Can you work these out from the drawing? Everything is in mm from the part's minimum corner. Round coordinates to 2 decimals unless told otherwise and drop trailing zeros. Write each loop counter-clockwise with the first axis right and the second up, starting at its lowest first coordinate (ties: lowest second). Pieces come first, ordered by that corner, then holes. Notation, with made-up numbers: (21, 60) -> (52, 60) arc R26 cw to (52, 78) -> close; hole circle Ø2 at (55.25, 25.5). An arc over 180 degrees is marked (long way). Answer as CSV lines item,"result".
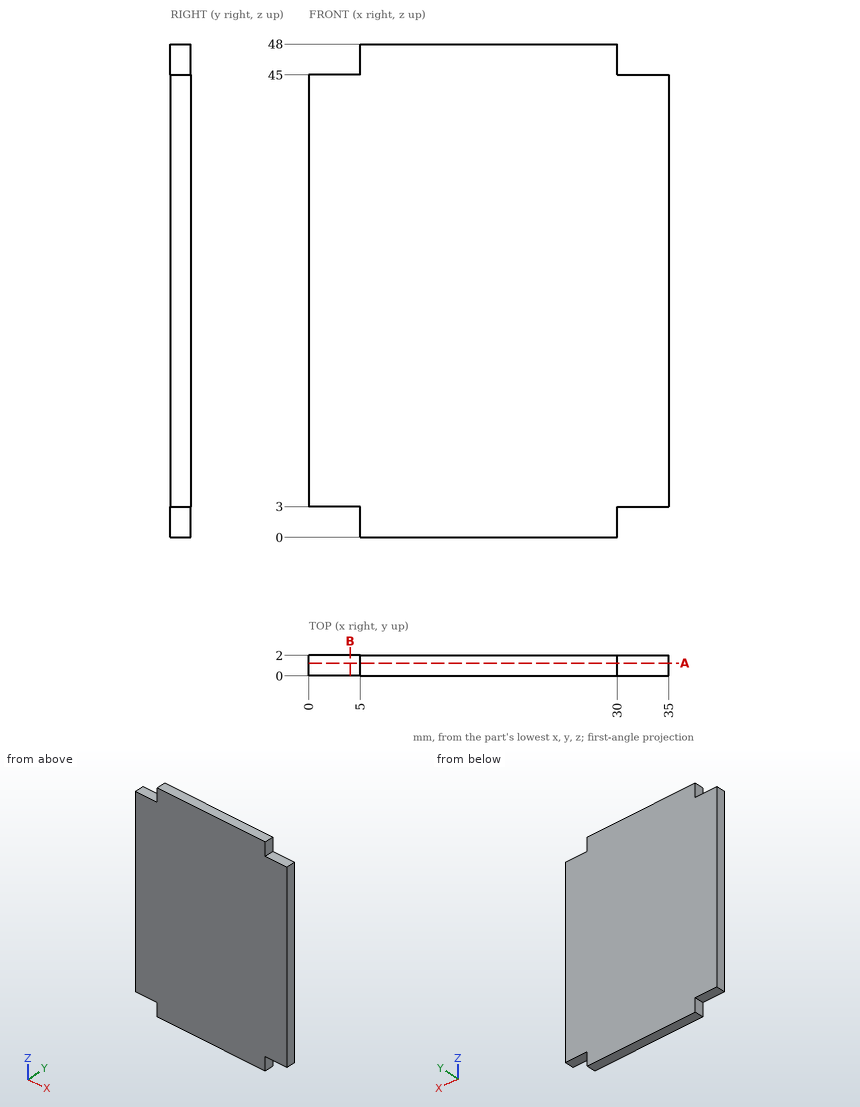
Item 1: Suppose I cut it at B-B, the plane x = 4. List the corners of the cut face in (y, z) for me, then the cut area to 3 significant figures.
Results found:
outline,"(0, 3) -> (2, 3) -> (2, 45) -> (0, 45) -> close"
area,"84.0 mm²"
Item 2: I need wall thicknesses on L1, parallel to Z at x = 31, y = 1.1; L2, parallel to X at y = 0.15, z = 2. Which ranges of each line are inside material? Lowest first, please.
Results found:
L1,"z = 3 to 45"
L2,"x = 5 to 30"
Item 3: Suppose I cut it at A-A, the plane y = 1.25. List the corners of the cut face in (x, z) for me, then the cut area to 3 significant figures.
Results found:
outline,"(0, 3) -> (5, 3) -> (5, 0) -> (30, 0) -> (30, 3) -> (35, 3) -> (35, 45) -> (30, 45) -> (30, 48) -> (5, 48) -> (5, 45) -> (0, 45) -> close"
area,"1,620 mm²"
Item 4: Will these pins go through, and if not, where does the flat tip stop? pin 1 (5 mm diameter, centred on x = 7, z = 29.5, fed in from -Y); pin 2 (0.6 mm diameter, centred on y = 1, z = 1, fed in from -X); pin 3 (1 mm diameter, centred on x = 3, y = 1.5, fed in from -Z); pin 4 (1 mm diameter, centred on y = 1.5, z = 1.5, fed in from +X).
Results found:
pin 1,"stops at y = 0"
pin 2,"stops at x = 5"
pin 3,"stops at z = 3"
pin 4,"stops at x = 30"
